Build history of the part. All positions in model axes, mm. Face numbers are marked on the shaded views. A direction names the side the tool comes from. Coordinates: 2 decimals unless noted, no trailing zeros. Loops run counter-clockwise (first coordinate to the right, second up) from the corner with the lowest first, then second, coordinate; pieces in that order, holes last.
(1) Two-plate mould, pull along Y, no slides. Class the marked faces 1, 2, 3 and 4: pulls with the +Y half, pulls with the -Y half, needs draft (parallel to the pull), parting line crosses it, or undercut.
(2) Flat gauge pins, fed straight in: P1, Ø12, axis at x = 34.5, z = 14.5, coming from the +Y side; P2, Ø1.5, axis at x = 32.5, z = 20.5, coming from the +Y side; P3, Ø2, axis at x = 29, z = 18, coming from the -Y side; P4, Ø4, axis at y = 10.5, z = -15.5, coming from the -X side. Where does each tip first touch, or does it go through?
(3) Slice it at C-C (y = 12). Give the cut face in (x, z), and give its area (3 significant figures).
(4) Slice it at D-D (x = 73). Give the number of separate pieces and of enclosed holes in the cut face, and give its area (3 significant figures).
(5) Tool access for the marked faces 5 and 6: list every direction of +Z, -Z, +X, -X, +Y, -Y with a clear straight run to the whole face (end or side of a thin tool).
(6) Wall check: L1, parallel to Y at x = 10, z = 0.5; L2, parallel to Z at x = 43, y = 5; L3, parallel to Z at x = 68.5, y = -13. Give the ranges that are in metal, low to high.
(7) Slice it at B-B (z = -18.5). Give the cut face in (x, y).
(8) Slice it at A-A (z = 0). Give the cut face in (x, y) (3 decimals).
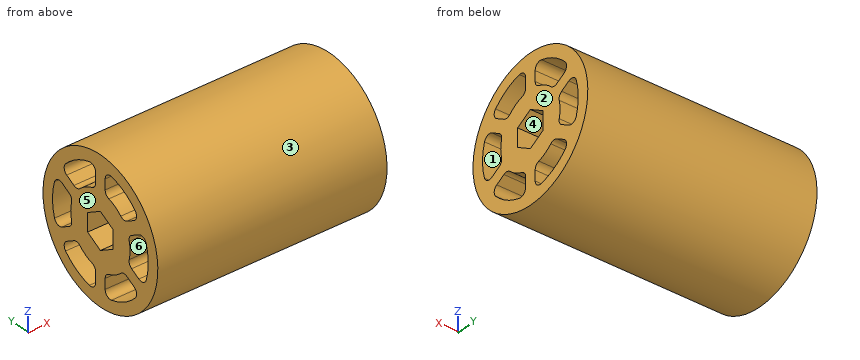
from build123d import *

# Parameters (mm, degrees)
CROQUIS1_R              = 28.575
SALIENTE_EXTRUIR1_DEPTH = 92.5
CORTAR_EXTRUIR1_DEPTH   = 101.942118315


with BuildPart() as part:
    # Croquis1 → Saliente-Extruir1 (new body)
    with BuildSketch(Plane(origin=(0, 0, 0), x_dir=(0, 0, -1), z_dir=(1, 0, 0))):
        Circle(CROQUIS1_R)
        Polygon((7.332348419, 0), (3.666174209, 6.35), (-3.666174209, 6.35), (-7.332348419, 0), (-3.666174209, -6.35), (3.666174209, -6.35), align=None, mode=Mode.SUBTRACT)
    extrude(amount=SALIENTE_EXTRUIR1_DEPTH)

    # Croquis2 → Cortar-Extruir1 (cut, through all)
    with BuildSketch(Plane(origin=(92.5, 0, 0), x_dir=(0, 0, -1), z_dir=(1, 0, 0))):
        with BuildLine():
            Line((-6.233796171, 15.550729765), (-8.292494443, 19.11649977))
            ThreePointArc((-8.292494443, 19.11649977), (-8.452873942, 21.324398032), (-6.820383997, 22.8195612))
            ThreePointArc((-6.820383997, 22.8195612), (0, 23.817682129), (6.820383997, 22.8195612))
            ThreePointArc((6.820383997, 22.8195612), (8.452873942, 21.324398032), (8.292494443, 19.11649977))
            Line((8.292494443, 19.11649977), (6.233796171, 15.550729765))
            ThreePointArc((6.233796171, 15.550729765), (5.037217596, 14.487169273), (3.442097, 14.350965426))
            ThreePointArc((3.442097, 14.350965426), (0, 14.758215751), (-3.442097, 14.350965426))
            ThreePointArc((-3.442097, 14.350965426), (-5.037136467, 14.487358051), (-6.233796171, 15.550729765))
        make_face()
        with BuildLine():
            Line((16.584225127, 2.376739002), (20.701621672, 2.376739002))
            ThreePointArc((20.701621672, 2.376739002), (22.693907405, 3.341795413), (23.172511718, 5.50315476))
            ThreePointArc((23.172511718, 5.50315476), (20.6267178, 11.90884103), (16.352127722, 17.31640637))
            ThreePointArc((16.352127722, 17.31640637), (14.241033463, 17.98260255), (12.409127229, 16.739760699))
            Line((12.409127229, 16.739760699), (10.350428956, 13.173990694))
            ThreePointArc((10.350428956, 13.173990694), (10.02785189, 11.605967133), (10.707252145, 10.156426122))
            ThreePointArc((10.707252145, 10.156426122), (12.780989772, 7.37910784), (14.149349145, 4.194539234))
            ThreePointArc((14.149349145, 4.194539234), (15.064865435, 2.881226199), (16.584225127, 2.376739002))
        make_face()
        with BuildLine():
            Line((10.350428935, -13.173990796), (12.409127207, -16.739760801))
            ThreePointArc((12.409127207, -16.739760801), (14.241033442, -17.982602652), (16.3521277, -17.316406472))
            ThreePointArc((16.3521277, -17.316406472), (20.626717779, -11.908841132), (23.172511697, -5.503154863))
            ThreePointArc((23.172511697, -5.503154863), (22.693907383, -3.341795515), (20.70162165, -2.376739104))
            Line((20.70162165, -2.376739104), (16.584225106, -2.376739104))
            ThreePointArc((16.584225106, -2.376739104), (15.064988336, -2.881390951), (14.149349124, -4.194539336))
            ThreePointArc((14.149349124, -4.194539336), (12.780989751, -7.379107943), (10.707252124, -10.156426225))
            ThreePointArc((10.707252124, -10.156426225), (10.027647818, -11.605943107), (10.350428935, -13.173990796))
        make_face()
        with BuildLine():
            Line((-6.233796214, -15.550729831), (-8.292494486, -19.116499836))
            ThreePointArc((-8.292494486, -19.116499836), (-8.452873985, -21.324398098), (-6.82038404, -22.819561265))
            ThreePointArc((-6.82038404, -22.819561265), (-4.3e-08, -23.817682194), (6.820383954, -22.819561265))
            ThreePointArc((6.820383954, -22.819561265), (8.452873899, -21.324398098), (8.2924944, -19.116499836))
            Line((8.2924944, -19.116499836), (6.233796128, -15.550729831))
            ThreePointArc((6.233796128, -15.550729831), (5.037136424, -14.487358117), (3.442096957, -14.350965491))
            ThreePointArc((3.442096957, -14.350965491), (-4.3e-08, -14.758215816), (-3.442097043, -14.350965491))
            ThreePointArc((-3.442097043, -14.350965491), (-5.037217639, -14.487169339), (-6.233796214, -15.550729831))
        make_face()
        with BuildLine():
            Line((-16.58422517, -2.376739067), (-20.701621714, -2.376739067))
            ThreePointArc((-20.701621714, -2.376739067), (-22.693907448, -3.341795478), (-23.172511761, -5.503154826))
            ThreePointArc((-23.172511761, -5.503154826), (-20.626717843, -11.908841095), (-16.352127764, -17.316406435))
            ThreePointArc((-16.352127764, -17.316406435), (-14.241033506, -17.982602615), (-12.409127271, -16.739760764))
            Line((-12.409127271, -16.739760764), (-10.350428999, -13.173990759))
            ThreePointArc((-10.350428999, -13.173990759), (-10.027851933, -11.605967199), (-10.707252188, -10.156426188))
            ThreePointArc((-10.707252188, -10.156426188), (-12.780989815, -7.379107906), (-14.149349188, -4.194539299))
            ThreePointArc((-14.149349188, -4.194539299), (-15.064865478, -2.881226264), (-16.58422517, -2.376739067))
        make_face()
        with BuildLine():
            Line((-10.350428978, 13.173990731), (-12.40912725, 16.739760736))
            ThreePointArc((-12.40912725, 16.739760736), (-14.241033484, 17.982602587), (-16.352127743, 17.316406407))
            ThreePointArc((-16.352127743, 17.316406407), (-20.626717822, 11.908841067), (-23.17251174, 5.503154797))
            ThreePointArc((-23.17251174, 5.503154797), (-22.693907426, 3.34179545), (-20.701621693, 2.376739039))
            Line((-20.701621693, 2.376739039), (-16.584225148, 2.376739039))
            ThreePointArc((-16.584225148, 2.376739039), (-15.064988378, 2.881390885), (-14.149349166, 4.194539271))
            ThreePointArc((-14.149349166, 4.194539271), (-12.780989794, 7.379107878), (-10.707252167, 10.156426159))
            ThreePointArc((-10.707252167, 10.156426159), (-10.027647861, 11.605943042), (-10.350428978, 13.173990731))
        make_face()
    extrude(amount=-CORTAR_EXTRUIR1_DEPTH, mode=Mode.SUBTRACT)


solid = part.part
Response values:
1. face 1: undercut
1. face 2: needs draft
1. face 3: parting line crosses it
1. face 4: undercut
2. P1: stops at y = 27.28
2. P2: stops at y = 20.65
2. P3: stops at y = -22.97
2. P4: passes through
3. outline: (0, -25.93) - (92.5, -25.93) - (92.5, -20.57) - (0, -20.57) - close; (0, -10.01) - (92.5, -10.01) - (92.5, 10.01) - (0, 10.01) - close; (0, 20.57) - (92.5, 20.57) - (92.5, 25.93) - (0, 25.93) - close
3. area: 2,840 mm2
4. separate pieces: 1
4. enclosed holes: 7
4. area: 1,620 mm2
5. face 5: +Z, -Z, -X, +Y, -Y
5. face 6: +X, -X
6. L1: y = -28.57 to -23.81, -14.75 to -6.35, 6.35 to 14.75, 23.81 to 28.57
6. L2: z = -28.13 to -23.24, -13.89 to -4.45, 4.45 to 13.89, 23.24 to 28.13
6. L3: z = -25.45 to -19.96, -10.26 to 10.26, 19.96 to 25.45
7. outline: (0, -21.78) - (92.5, -21.78) - (92.5, -15) - (0, -15) - close; (0, -2.38) - (92.5, -2.38) - (92.5, 2.38) - (0, 2.38) - close; (0, 15) - (92.5, 15) - (92.5, 21.78) - (0, 21.78) - close
8. outline: (0, -28.575) - (92.5, -28.575) - (92.5, -23.818) - (0, -23.818) - close; (0, -14.758) - (92.5, -14.758) - (92.5, -6.35) - (0, -6.35) - close; (0, 6.35) - (92.5, 6.35) - (92.5, 14.758) - (0, 14.758) - close; (0, 23.818) - (92.5, 23.818) - (92.5, 28.575) - (0, 28.575) - close
